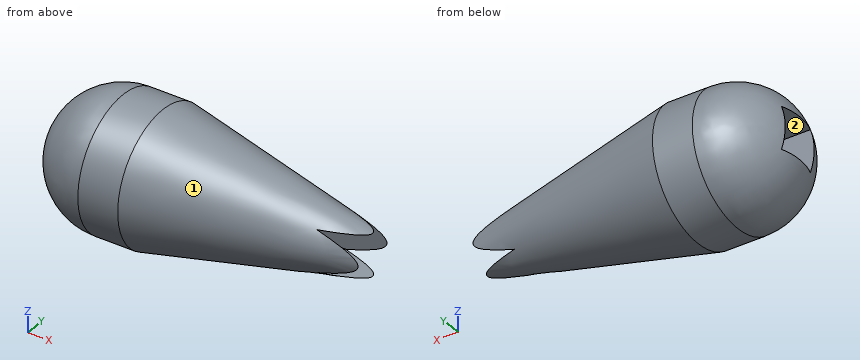
from build123d import *

# Parameters (mm, degrees)
F1_W     = 6.35
F1_H     = 6.35
F3_DEPTH = 62.406244


with BuildPart() as f2:
    # F0 (on Top) → F2 (revolve)
    with BuildSketch(Plane.XY):
        with BuildLine():
            Line((-9.333627, 1.915156), (-46.597632, 9.852656))
            Line((-46.597632, 9.852656), (-52.552588, 9.852656))
            ThreePointArc((-52.552588, 9.852656), (-59.519468, 6.96688), (-62.405244, 0))
            Line((-62.405244, 0), (-7.762354, 0))
            ThreePointArc((-7.762354, 0), (-8.212572, 1.232769), (-9.333627, 1.915156))
        make_face()
    revolve(axis=Axis((-35.677824, 0, 0), (1, 0, 0)))

    # F1 (on Right) → F3 (cut, through all)
    with BuildSketch(Plane.YZ):
        Rectangle(F1_W, F1_H)
    extrude(amount=-F3_DEPTH, mode=Mode.SUBTRACT)


solid = f2.part
Geometry: final body of the model. Coordinates: model frame, mm. Face numbers are marked on the shaded views. Give positions to 0.01 mm unless a question says otherwise; leave off trailing zeros. Write each loop counter-clockwise with the first axis right and the second up, starting at its lowest first coordinate (ties: lowest second). Pieces come first, ordered by that corner, then holes. Notation, with made-up numbers: (5, 16.5) - (44, 16.5) arc R23 ccw to (44, 28.5) - close; hole circle Ø5 at (7, 73.25). An arc over 180 degrees is marked (long way). Return JSON: item names as keys, results as strings. Group by question number.
1) Line query: line 1 (Z direction, x = -33.5, y = -1) (3 decimals); line 2 (Z direction, x = -35, y = -2.75) (3 decimals); line 3 (Y direction, x = -26.5, z = -2.5) (3 decimals). Output: solid intervals per line, ascending.
2) Mould query, pull axis Y, two halves, no side actions, for the marked faces 1 and 2. Classes: released by +Y, released by -Y, zero draft, split by the parting line, or undercut.
3) Section A-A on x = -36. Return the cut outline in (y, z) (3 decimals), plus the area to 3 significant figures.
4) First-contact query: P1, Ø1, axis at x = -48, y = -2.5, coming from the +Z side; P2, Ø7, axis at x = -34, y = -1, coming from the +Z side; P3, Ø5, axis at x = -43, z = -3, coming from the -Y side. Flat tips, straight axial feed; report the tip coordinate or a pass-through.
Filled in:
{
 "1": {"line 1": "z = -6.992 to -3.175, 3.175 to 6.992", "line 2": "z = -6.851 to -3.175, 3.175 to 6.851", "line 3": "y = -4.979 to -3.175, 3.175 to 4.979"},
 "2": {"face 1": "split by the parting line", "face 2": "undercut"},
 "3": {"outline": "circle Ø15.191 at (0, 0); hole (-3.175, -3.175) - (3.175, -3.175) - (3.175, 3.175) - (-3.175, 3.175) - close", "area": "141 mm^2"},
 "4": {"P1": "stops at z = 9.65", "P2": "stops at z = 7.89", "P3": "stops at y = -9.39"}
}
